Read the model definition and answer for the solid it produces. Units are mm, in the model's axes. Face numbers are marked on the shaded views. A direction names the side the tool comes from. Give positions to 0.01 mm unless a question says otherwise; leave off trailing zeros. Order: outer loops, then holes, each group sorted by start corner. A loop starts at its lowest first (then second) coordinate and runs counter-clockwise, first axis right, second up. Notation, with made-up numbers: (-18.5, 45) -> (28.5, 45) arc R34 cw to (28.5, 82) -> close; hole circle Ø5 at (66, 3.25). An arc over 180 degrees is marked (long way). Use one line per item in the form item = value.
```python
from build123d import *

# Parameters (mm, degrees)
F0_R      = 15
F1_DEPTH  = 5
F1_TAPER  = 20
F1_FACE_R = 13.1801488287
F2_DEPTH  = 10
F2_TAPER  = 5
F2_FACE_R = 12.3052621934
F3_DEPTH  = 10
F3_TAPER  = 3
F3_FACE_R = 11.7811844006
F4_DEPTH  = 10
F4_TAPER  = -3
F4_FACE_R = 12.3052621934
F5_DEPTH  = 10
F5_TAPER  = -5
F5_FACE_R = 13.1801488287
F6_DEPTH  = 5
F6_TAPER  = -20
F7_R      = 10.38
F8_DEPTH  = 47


with BuildPart() as f1:
    # F0 (on Top) → F1 (new body)
    with BuildSketch(Plane.XY):
        Circle(F0_R)
    extrude(amount=F1_DEPTH, taper=F1_TAPER)

    # F1_face (on face) → F2 (join)
    with BuildSketch(Plane.XY.offset(5)):
        Circle(F1_FACE_R)
    extrude(amount=F2_DEPTH, taper=F2_TAPER)

    # F2_face (on face) → F3 (join)
    with BuildSketch(Plane.XY.offset(15)):
        Circle(F2_FACE_R)
    extrude(amount=F3_DEPTH, taper=F3_TAPER)

    # F3_face (on face) → F4 (join)
    with BuildSketch(Plane.XY.offset(25)):
        Circle(F3_FACE_R)
    extrude(amount=F4_DEPTH, taper=F4_TAPER)

    # F4_face (on face) → F5 (join)
    with BuildSketch(Plane.XY.offset(35)):
        Circle(F4_FACE_R)
    extrude(amount=F5_DEPTH, taper=F5_TAPER)

    # F5_face (on face) → F6 (join)
    with BuildSketch(Plane.XY.offset(45)):
        Circle(F5_FACE_R)
    extrude(amount=F6_DEPTH, taper=F6_TAPER)

    # F7 (on face) → F8 (cut)
    with BuildSketch(Plane.XY.offset(50)):
        Circle(F7_R)
    extrude(amount=-F8_DEPTH, mode=Mode.SUBTRACT)


solid = f1.part
```
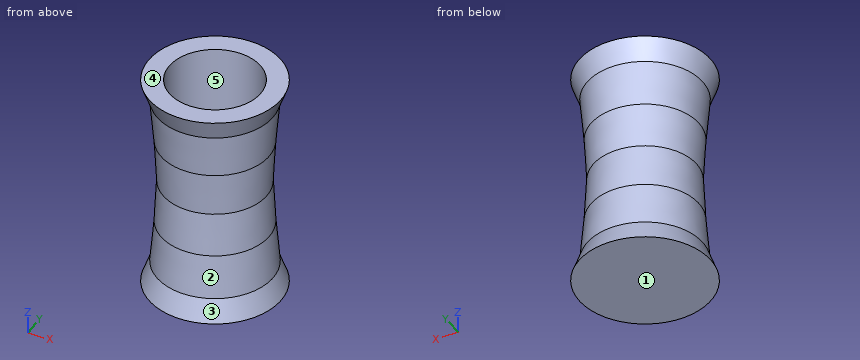
Item 1: The part is cut by section C-C on z = 34. Give the vertices of the cut face in (x, y), and give its area (3 significant figures).
Checks:
outline = circle Ø24.51 at (0, 0); hole circle Ø20.76 at (0, 0)
area = 133 mm²
Item 2: Given pin 1 Ø6 at (y, z) = (-2, 33) entering from -X; pin 2 Ø5 at (y, z) = (-4.5, 20.5) entering from +X; pin 3 Ø3 at (x, z) = (9, 26.5) entering from -Y, each flat-ended and moving along its own axis, determine where each tip first touches the part or whether it passes through.
Checks:
pin_1 = -12.35
pin_2 = 11.87
pin_3 = -9.19
Item 3: The part is cut by section B-B on z = 40. Give the vertices of the cut face in (x, y), and give its area (3 significant figures).
Checks:
outline = circle Ø25.49 at (0, 0); hole circle Ø20.76 at (0, 0)
area = 172 mm²
Item 4: Straight lines are drawn through the part: L1, parallel to Z at x = -7, y = 3; L2, parallel to Y at x = 4.5, z = 48.5; L3, parallel to Z at x = -10.5, y = 9. For each, find the intervals that lie inside material, in ascending order. Write a range as from..to.
Checks:
L1 = 0..3
L2 = -13.74..-9.35, 9.35..13.74
L3 = 0..3.22, 46.78..50
Item 5: Determine the mould class of the marked faces 3, 4 and 5 for opening direction Y: +Y half, -Y half, draft (parallel to the pull), parting line (faces both ways), or undercut.
Checks:
face_3 = parting line
face_4 = draft
face_5 = undercut
Item 6: The part is cut by section A-A on x = 0. Give the vertices of the cut face in (y, z), and give its area (3 significant figures).
Checks:
outline = (-15, 0) -> (15, 0) -> (13.18, 5) -> (12.31, 15) -> (11.78, 25) -> (12.31, 35) -> (13.18, 45) -> (15, 50) -> (10.38, 50) -> (10.38, 3) -> (-10.38, 3) -> (-10.38, 50) -> (-15, 50) -> (-13.18, 45) -> (-12.31, 35) -> (-11.78, 25) -> (-12.31, 15) -> (-13.18, 5) -> close
area = 298 mm²
Item 7: Which of the six approach directions +Z, -Z, +X, -X, +Y, -Y give full straight-line access (tool end or side, diameter ignored) to the marked faces 1 and 2?
Checks:
face_1 = -Z, +X, -X, +Y, -Y
face_2 = none
